Autodesk Inventor part; units mm, degrees
ref_plane "YZ Plane" through (0, 0, 0) normal (1, 0, 0) x (0, 1, 0)
ref_plane "XZ Plane" through (0, 0, 0) normal (0, 1, 0) x (-1, 0, 0)
ref_plane "XY Plane" through (0, 0, 0) normal (0, 0, 1) x (1, 0, 0)
sketch "Эскиз1" plane through (0, 0, 0) normal (0, 0, 1) x (1, 0, 0)
  circle A0 centre (0, 0) radius 32
  circle A1 centre (0, 0) radius 100
  dimension "d0" = 64
  dimension "d1" = 200
extrude "Выдавливание1" add sketch "Эскиз1" along normal blind 10
sketch "Эскиз2" plane through (0, 0, 10) normal (0, 0, 1) x (1, 0, 0)
  circle A0 centre (0, 0) radius 100
  circle A1 centre (0, 0) radius 70
  dimension "d4" = 140
extrude "Выдавливание2" add sketch "Эскиз2" along normal blind 5.5
sketch "Эскиз3" plane through (0, 0, 0) normal (0, 0, -1) x (-1, 0, 0)
  line L0 (0, 0) -> (78.5298, 32.5281)
  line L1 (140, 0) -> (-140, 0)
  dimension "d8" = 85
  dimension "d9" = 22.5
hole "Отверстие1" at (-78.5298, 32.5281, 0) direction (0, 0, 1) diameter 12 end through all
pattern_circular "Круговой массив1" count 8 over 360 about axis through (0, 0, 0) along (0, 0, 1) of "Отверстие1"
chamfer "Фаска1" distance 2 angle 45 3 edges at (-32, 0, 0) (-32, 0, 10) (-70, 0, 15.5)
fillet "Сопряжение1" radius 2 1 edges at (-70, 0, 10)
sketch "Эскиз4" plane through (0, 0, 15.5) normal (0, 0, 1) x (1, 0, 0)
  circle A0 centre (0, 0) radius 72
  circle A1 centre (0, 0) radius 100
  line L0 (17.039, -69.9548) -> (17.039, -98.5377)
  circle A2 centre (0, 0) radius 100
  line L1 (0, -140) -> (0, 140)
  line L2 (-17.039, -69.9548) -> (-17.039, -98.5377)
  line L3 (-17.039, -69.9548) -> (-17.039, -65.8306)
  circle A3 centre (0, 0) radius 68
  line L4 (17.039, -69.9548) -> (17.039, -65.8306)
extrude "Выдавливание3" cut sketch "Эскиз4" against normal blind 7 contours L0 A1 L1 A0 | A0 L1 A3 L4 | L1 A1 L2 A0 | A0 L3 A3 L1 picked at (9.5127, -80.7365) picked at (15.1684, -67.6061) picked at (-9.5127, -80.7365) picked at (-15.1684, -67.6061)
properties part number "Крышка перегородки22" material "Чугун, серый"
Input: part model. Units: mm. Frame: model coordinates. A direction names the side the tool comes from. Coordinates: 2 decimals unless noted, no trailing zeros. Order: outer loops, then holes, each group sorted by start corner. A loop starts at its lowest first (then second) coordinate and runs counter-clockwise, first axis right, second up. Notation, with made-up numbers: M -22,15 L -12,15 A32 cw -12,42 Z; hole C -22,83 d8. An arc over 180 degrees is marked long. Answer as CSV lines item,"result".
1. Pull-direction query (Y, two-part tool) for faces 4 (the flat face through (-1, -43, 0)), 5 (the cylindrical face through (-26.984, 80.824, 7.858)); classes: released by +Y, released by -Y, zero draft, split by the parting line, or undercut.
Reported:
face 4,"zero draft"
face 5,"undercut"
2. First-contact query: P1, Ø3, axis at y = 67, z = 6, coming from the -X side; P2, Ø7.5, axis at y = -85.5, z = 13.5, coming from the -X side; P3, Ø5.5, axis at y = -80.5, z = 13.5, coming from the +X side. Flat tips, straight axial feed; report the tip coordinate or a pass-through.
Reported:
P1,"x = -75.56"
P2,"x = -57.59"
P3,"x = 62.89"
3. Material intervals for line 1 (Y direction, x = 75.5, z = 0.5); line 2 (X direction, y = 77, z = 8.75); line 3 (Y direction, x = 27, z = 14.5), sorted ascending. Write a range as from..to.
Reported:
line 1,"-65.57..-37.71, -27.35..27.35, 37.71..65.57"
line 2,"-63.8..-38.33, -26.73..26.73, 38.33..63.8"
line 3,"-96.29..-80.86, -76.2..-65.67, 65.67..76.2, 80.86..96.29"
4. Section A-A (y = 0). Return the cut outline in (x, z), then the cut area to 3 significant figures.
Reported:
outline,"M -100,0 L -34,0 L -32,2 L -32,8 L -34,10 L -68,10 A2 cw -70,12 L -70,13.5 L -72,15.5 L -100,15.5 Z; M 32,2 L 34,0 L 100,0 L 100,15.5 L 72,15.5 L 70,13.5 L 70,12 A2 cw 68,10 L 34,10 L 32,8 Z"
area,"1,680 mm2"
5. Access query for faces 1 (the flat face through (14.2, 31.2, 10)), 2 (the cylindrical face through (-6.94, 31.24, 4.96)), 3 (the flat face through (0, -83, 8.5)). Directions: +Z, -Z, +X, -X, +Y, -Y. A direction counts if a zero-diameter tool reaches every point of the face in a straight line with its end or side. Return the directions, or none.
Reported:
face 1,"+Z"
face 2,"+Z, -Z"
face 3,"+Z, -Y"
6. Section B-B (x = 0). Return the cut outline in (y, z), then the cut area to 3 significant figures.
Reported:
outline,"M -100,0 L -34,0 L -32,2 L -32,8 L -34,10 L -68,10 L -68,8.5 L -100,8.5 Z; M 32,2 L 34,0 L 100,0 L 100,15.5 L 72,15.5 L 70,13.5 L 70,12 A2 cw 68,10 L 34,10 L 32,8 Z"
area,"1,470 mm2"
